Model file for the job. Use its own axes, mm. Round coordinates to 2 decimals unless told otherwise and drop trailing zeros. Loops run counter-clockwise (first coordinate to the right, second up) from the corner with the lowest first, then second, coordinate; pieces in that order, holes last. Notation, with made-up numbers: M -17.5,-26 L 23.5,-26 A19 ccw 23.5,-16 Z; hole C -9,24 d3. An arc over 180 degrees is marked long. Use a Markdown table: item, result. Add a question column.
Q1. Probe line 1 (Z direction, x = -17, y = 6.35); line 2 (X direction, y = 4.75, z = 16.5); line 3 (Z direction, x = -18, y = 6.35). List the from-to ranges inside material, lowest first. Write a range as from..to.
Q2. Cut at A-A (z = 294.5). Give the cut face in (x, y).
Q3. Pin check, flat tips, straight feed: pin 1 (1.5 mm diameter, centred on y = 8.5, z = 340, fed in from -X); pin 2 (4 mm diameter, centred on y = 8, z = 342, fed in from +X); pin 3 (3 mm diameter, centred on y = 6.35, z = 88.9, fed in from +X). Stop position of each tip, or through.
from build123d import *

# Parameters (mm, degrees)
F0_W     = 63.5
F0_H     = 12.7
F1_DEPTH = 381
F3_D     = 5.1054
F3_DEPTH = 19.05
F3_TIP   = 1.5338169022
F4_W     = 50.8
F4_H     = 31.75
F5_DEPTH = 6.35
F7_D     = 3.7973
F7_DEPTH = 19.05
F7_START = 6.35
F7_TIP   = 1.1408240143
F8_SIZE2 = 38.1
F8_SIZE  = 203.2
F9_R     = 19.05


with BuildPart() as f1:
    # F0 (on Top) → F1 (new body)
    with BuildSketch(Plane.XY):
        with Locations((-31.75, 6.35)):
            Rectangle(F0_W, F0_H)
    extrude(amount=F1_DEPTH)

    # F3
    with Locations(Plane(origin=(0, 0, 0), x_dir=(1, 0, 0), z_dir=(0, 0, -1))):
        with Locations((-15.875, -6.35), (-53.975, -6.35)):
            Hole(F3_D / 2, depth=F3_DEPTH)
            with Locations((0, 0, -(F3_DEPTH + F3_TIP / 2))):  # 118° drill point
                Cone(0, F3_D / 2, F3_TIP, mode=Mode.SUBTRACT)

    # F4 (on face) → F5 (cut)
    with BuildSketch(Plane.YZ):
        with Locations((25.4, 79.375)):
            Rectangle(F4_W, F4_H)
        with Locations((25.4, 339.725)):
            Rectangle(F4_W, F4_H)
    extrude(amount=-F5_DEPTH, mode=Mode.SUBTRACT)

    # F7
    # its depths count from where the whole tool has entered the part; down to there all is cleared
    with Locations(Plane.YZ.offset(-F7_START)):
        with Locations((6.35, 69.85), (6.35, 88.9), (6.35, 330.2), (6.35, 349.25)):
            Hole(F7_D / 2, depth=F7_DEPTH)
            with Locations((0, 0, -(F7_DEPTH + F7_TIP / 2))):  # 118° drill point
                Cone(0, F7_D / 2, F7_TIP, mode=Mode.SUBTRACT)

    # F8
    f8_edges = [f1.edges().sort_by_distance(p)[0] for p in [
        (-63.5, 6.35, 381),
    ]]
    f8_side = f1.faces().sort_by_distance((-63.5, 6.35, 190.5))[0]
    chamfer(f8_edges, length=F8_SIZE, length2=F8_SIZE2, reference=f8_side)

    # F9
    f9_edges = [f1.edges().sort_by_distance(p)[0] for p in [
        (-25.4, 6.35, 381),
        (-63.5, 6.35, 177.8),
    ]]
    fillet(f9_edges, radius=F9_R)


solid = f1.part
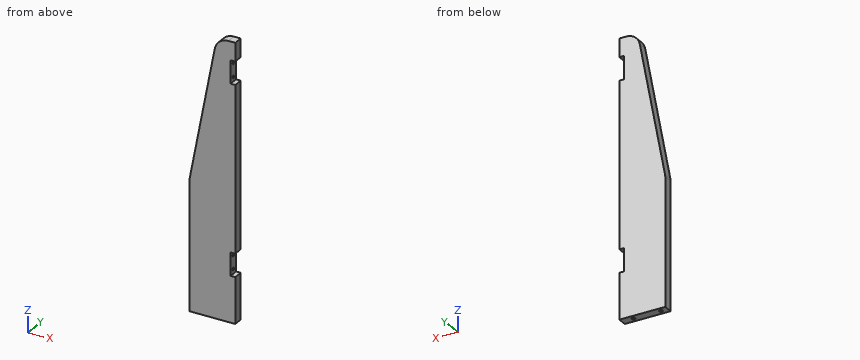
Checked values:
| question | item | result |
|---|---|---|
| 1 | line 1 | z = 19.91..67.95, 71.75..87, 90.8..328.3, 332.1..347.35, 351.15..379.5 |
| 1 | line 2 | x = -63.5..-55.96, -51.99..-17.86, -13.89..0 |
| 1 | line 3 | z = 19.31..67.95, 71.75..87, 90.8..328.3, 332.1..347.35, 351.15..379.04 |
| 2 | outline | M -41.62,0 L 0,0 L 0,12.7 L -41.62,12.7 Z |
| 3 | pin 1 | stops at x = -33.23 |
| 3 | pin 2 | stops at x = -6.35 |
| 3 | pin 3 | stops at x = -25.64 |
